CAD build for the part. Positions are in the model's coordinates, mm. A direction names the side the tool comes from. Give positions to 0.01 mm unless a question says otherwise; leave off trailing zeros. Loops run counter-clockwise (first coordinate to the right, second up) from the corner with the lowest first, then second, coordinate; pieces in that order, holes last. Notation, with made-up numbers: M 16.5,36 L 41.5,36 A20 cw 41.5,52 Z; hole C 39,27.5 d4. An arc over 180 degrees is marked long. Answer as CSV lines item,"result".
from build123d import *

# Parameters (mm, degrees)
F1_DEPTH = 27.5
F2_W     = 20
F2_H     = 2
F3_DEPTH = 120
F4_W     = 4
F4_H     = 22
F5_DEPTH = 15
F6_SIZE2 = 14.0041507642
F6_SIZE  = 20
F8_DEPTH = 15
F9_SIZE2 = 20
F9_SIZE  = 14.0041507642
F10_F1_R = 1.5
F10_F2_R = 1.5
F10_F3_R = 1.5
F10_F4_R = 1.5
F10_F5_R = 1.5
F10_F6_R = 1.5
F10_F7_R = 1.5
F10_F8_R = 1.5


# Not quite as in the source:
# - a feature names something its author has since deleted; it is built from what else it names


with BuildPart() as f1:
    # F0 (on Top) → F1 (new body, symmetric)
    with BuildSketch(Plane.XY):
        with BuildLine():
            Line((-10, -15.9872266478), (0, -15.9872266478))
            Line((0, -15.9872266478), (10, -15.9872266478))
            ThreePointArc((10, -15.9872266478), (20.5, -5.4872266478), (10, 5.0127733522))
            Line((10, 5.0127733522), (0, 5.0127733522))
            Line((0, 5.0127733522), (-10, 5.0127733522))
            ThreePointArc((-10, 5.0127733522), (-20.5, -5.4872266478), (-10, -15.9872266478))
        make_face()
        with BuildLine():
            Line((0, 3.0127733522), (10, 3.0127733522))
            ThreePointArc((10, 3.0127733522), (18.5, -5.4872266478), (10, -13.9872266478))
            Line((10, -13.9872266478), (0, -13.9872266478))
            Line((0, -13.9872266478), (-10, -13.9872266478))
            ThreePointArc((-10, -13.9872266478), (-18.5, -5.4872266478), (-10, 3.0127733522))
            Line((-10, 3.0127733522), (0, 3.0127733522))
        make_face(mode=Mode.SUBTRACT)
    extrude(amount=F1_DEPTH, both=True)

    # F2 (on face) → F3 (join)
    with BuildSketch(Plane(origin=(0, -13.9872266478, 0), x_dir=(-1, 0, 0), z_dir=(0, 1, 0))):
        with Locations((0, -4.5)):
            Rectangle(F2_W, F2_H)
        with BuildLine():
            ThreePointArc((-15.5, 0), (-13.8890872965, -3.8890872965), (-10, -5.5))
            Line((-10, -5.5), (-10, -3.5))
            ThreePointArc((-10, -3.5), (-12.4748737342, -2.4748737342), (-13.5, 0))
            ThreePointArc((-13.5, 0), (-12.4748737342, 2.4748737342), (-10, 3.5))
            Line((-10, 3.5), (-10, 5.5))
            ThreePointArc((-10, 5.5), (-13.8890872965, 3.8890872965), (-15.5, 0))
        make_face()
        with BuildLine():
            Line((10, -3.5), (10, -5.5))
            ThreePointArc((10, -5.5), (13.8890872965, -3.8890872965), (15.5, 0))
            ThreePointArc((15.5, 0), (13.8890872965, 3.8890872965), (10, 5.5))
            Line((10, 5.5), (10, 3.5))
            ThreePointArc((10, 3.5), (12.4748737342, 2.4748737342), (13.5, 0))
            ThreePointArc((13.5, 0), (12.4748737342, -2.4748737342), (10, -3.5))
        make_face()
        with Locations((0, 4.5)):
            Rectangle(F2_W, F2_H)
    extrude(amount=-F3_DEPTH)

    # F4 (on face) → F5 (join)
    with BuildSketch(Plane.XZ.offset(15.9872266478)):
        with Locations((0, 16.5)):
            Rectangle(F4_W, F4_H)
    extrude(amount=F5_DEPTH)

    # F6
    f6_edges = [f1.edges().sort_by_distance(p)[0] for p in [
        (0, -30.987227, 27.5),
    ]]
    f6_side = f1.faces().sort_by_distance((0, -30.987227, 16.5))[0]
    chamfer(f6_edges, length=F6_SIZE, length2=F6_SIZE2, reference=f6_side)

    # F7 (on face) → F8 (join)
    with BuildSketch(Plane.XZ.offset(15.9872266478)):
        Polygon((1.9211450554, -5.5), (0, -5.5), (-2.0788549446, -5.5), (-2.0788549446, -27.5), (1.9211450554, -27.5), align=None)
    extrude(amount=F8_DEPTH)

    # F9
    f9_edges = [f1.edges().sort_by_distance(p)[0] for p in [
        (-0.078855, -30.987227, -27.5),
    ]]
    f9_side = f1.faces().sort_by_distance((-6.039427, -15.441608, -27.5))[0]
    chamfer(f9_edges, length=F9_SIZE, length2=F9_SIZE2, reference=f9_side)

    # F10: fillet of radius 1.5 on 12 edges, made by hand

    # F10_f1
    f10_f1_edges = [f1.edges().sort_by_distance(p)[0] for p in [
        (-2.0788549446, -15.9872266478, -16.5),
    ]]
    fillet(f10_f1_edges, radius=F10_F1_R)

    # F10_f2
    f10_f2_edges = [f1.edges().sort_by_distance(p)[0] for p in [
        (-2.0788549446, -24.2372266478, -5.5),
    ]]
    fillet(f10_f2_edges, radius=F10_F2_R)

    # F10_f3
    f10_f3_edges = [f1.edges().sort_by_distance(p)[0] for p in [
        (1.9211450554, -15.9872266478, -16.5),
    ]]
    fillet(f10_f3_edges, radius=F10_F3_R)

    # F10_f4
    f10_f4_edges = [f1.edges().sort_by_distance(p)[0] for p in [
        (1.9211450554, -24.2372266478, -5.5),
    ]]
    fillet(f10_f4_edges, radius=F10_F4_R)

    # F10_f5
    f10_f5_edges = [f1.edges().sort_by_distance(p)[0] for p in [
        (-0.0788549446, -30.9872266478, -5.5),
    ]]
    fillet(f10_f5_edges, radius=F10_F5_R)

    # F10_f6
    f10_f6_edges = [f1.edges().sort_by_distance(p)[0] for p in [
        (-2, -15.9872266478, 17.25),
    ]]
    fillet(f10_f6_edges, radius=F10_F6_R)

    # F10_f7
    f10_f7_edges = [f1.edges().sort_by_distance(p)[0] for p in [
        (2, -15.9872266478, 17.25),
    ]]
    fillet(f10_f7_edges, radius=F10_F7_R)

    # F10_f8
    f10_f8_edges = [f1.edges().sort_by_distance(p)[0] for p in [
        (0, -30.9872266478, 5.5),
    ]]
    fillet(f10_f8_edges, radius=F10_F8_R)


solid = f1.part
1) Flat gauge pins, fed straight in: pin 1 (10 mm diameter, centred on x = -11.5, y = -40, fed in from -Z); pin 2 (1.5 mm diameter, centred on y = -20.5, z = 7.5, fed in from -X); pin 3 (2 mm diameter, centred on x = 5, z = 21.5, fed in from -Y). Where does each tip first touch, or does it go through?
Answer below:
pin 1,"stops at z = -5.5"
pin 2,"stops at x = -2.02"
pin 3,"stops at y = -15.99"
2) Band-saw the part on C-C on z = 14. Give the cut face in (x, y), and give its area (3 significant figures).
Answer below:
outline,"M -10,-15.99 L -3.5,-15.99 A1.5 cw -2,-17.49 L -2,-26.44 L 2,-26.44 L 2,-17.49 A1.5 cw 3.5,-15.99 L 10,-15.99 A10.5 ccw 10,5.01 L -10,5.01 A10.5 ccw Z; hole M -10,-13.99 L 10,-13.99 A8.5 ccw 10,3.01 L -10,3.01 A8.5 ccw Z"
area,"242 mm^2"
3) Which spindle directions (+Z, -Z, +X, -X, +Y, -Y) get a long thin tool onto all of the face, cutting with end or side? Do faces 1 (the face through (-7, -15.987, -17)), 2 (the face through (2, -23, 15)), 3 (the face through (0, -74, 3.5)), 4 (the face through (-7, -15.987, 17)), 5 (the face through (18.498, -5.3, 0.385)). Say none if no direction does.
Answer below:
face 1,"-Z, -X, -Y"
face 2,"+Z, +X, -Y"
face 3,"-Y"
face 4,"+Z, -X, -Y"
face 5,"+Z, -Z"
4) Band-saw the part on A-A on y = -63. Give the cut face in (x, z).
Answer below:
outline,"M -10,-5.5 L 10,-5.5 A5.5 ccw 10,5.5 L -10,5.5 A5.5 ccw Z; hole M -10,-3.5 L 10,-3.5 A3.5 ccw 10,3.5 L -10,3.5 A3.5 ccw Z"
5) Band-saw the part on B-B on z = -19. Give the cut face in (x, y), and give its area (3 significant figures).
Answer below:
outline,"M -10,-15.99 L -3.58,-15.99 A1.5 cw -2.08,-17.49 L -2.08,-22.93 L 1.92,-22.93 L 1.92,-17.49 A1.5 cw 3.42,-15.99 L 10,-15.99 A10.5 ccw 10,5.01 L -10,5.01 A10.5 ccw Z; hole M -10,-13.99 L 10,-13.99 A8.5 ccw 10,3.01 L -10,3.01 A8.5 ccw Z"
area,"228 mm^2"
6) Mould opens along X. For faces 6 (the face through (0, -15.987, 0)), 7 (the face through (-20.5, -5.3, 0.4)), 8 (the face through (-0.029, -23.887, 17.64)) say: +X half, -X half, draft (parallel to the pull), parting line (faces both ways), or undercut.
Answer below:
face 6,"undercut"
face 7,"-X half"
face 8,"draft"
7) Band-saw the part on D-D on y = -21.5. Give the cut face in (x, z).
Answer below:
outline,"M -10,-5.5 L -3.58,-5.5 A1.5 cw -2.08,-7 L -2.08,-21.05 L 1.92,-21.05 L 1.92,-7 A1.5 cw 3.42,-5.5 L 10,-5.5 A5.5 ccw 10,5.5 L 3.5,5.5 A1.5 cw 2,7 L 2,21.05 L -2,21.05 L -2,7 A1.5 cw -3.5,5.5 L -10,5.5 A5.5 ccw Z; hole M -10,-3.5 L 10,-3.5 A3.5 ccw 10,3.5 L -10,3.5 A3.5 ccw Z"
8) Drill centre lines: line 1 (Z direction, x = 6.5, y = -71); line 2 (Y direction, x = -4, z = -23); line 3 (Y direction, x = -13.5, z = 13). Where is each one in solid material? Low to high. Write a range as from..to.
Answer below:
line 1,"z = -5.5..-3.5, 3.5..5.5"
line 2,"y = -15.99..-13.99, 3.01..5.01"
line 3,"y = -15.39..-13.23, 2.26..4.41"
